Could you check a few things on this model? Use its own coordinates, in mm. A direction names the side the tool comes from. Give positions to 0.01 mm unless a question says otherwise; leave off trailing zeros. Order: outer loops, then holes, each group sorted by start corner. A loop starts at its lowest first (then second) coordinate and runs counter-clockwise, first axis right, second up.
(1) Imagine slicing it at B-B, the plane y = 9.5. Write out the boundary of the cut face in (x, z), then the cut area to 3 significant figures.
(2) If we mould it in two halves opening along Y, with no side actions, what happens to faces 4 (the flat face through (22, -0.8, -3)), 5 (the flat face through (22, 0, -3)), 6 (the flat face through (22, 25, 0.8)), 7 (the flat face through (22, 50, -3))? For each: released by +Y, released by -Y, zero draft, split by the parting line, or undercut.
(3) If I drill on probe 1 along X at (y, z) = (32.5, -3.05); probe 2 along X at (y, z) = (17, -0.4); probe 3 along Y at (x, z) = (36, -1.8), over which ranges is the centre line in solid material (lowest first)?
(4) Will this pin go through, and if not, where does the flat tip stop? pin 1 (1 mm diameter, centred on x = 27, y = 7.5, fed in from -Z).
(5) Imagine slicing it at A-A, the plane z = -2.5. Write out the boundary of the cut face in (x, y).
(6) On a 3-axis mill with a long thin cutter (end or side, diameter ignored), from which of +Z, -Z, +X, -X, +Y, -Y can I reach the whole of each face in a straight line? I mean faces 1 (the flat face through (45.8, 25, -3)), 2 (the cylindrical face through (33.5, 50.4, -3.1)), 3 (the flat face through (45, 25, -3)). Say none if no direction works.
(7) Imagine slicing it at C-C, the plane x = 33.5. Write out the boundary of the cut face in (y, z), then the cut area to 3 significant figures.
from build123d import *

# Parameters (mm, degrees)
F0_W     = 46.6
F0_H     = 51.6
F0_W_2   = 45
F0_H_2   = 50
F1_DEPTH = 0.8
F2_DEPTH = 5
F4_DEPTH = 0.8
F5_R     = 1


with BuildPart() as f1:
    # F0 (on Top) → F1 (new body)
    with BuildSketch(Plane.XY):
        with Locations((22.5, 25)):
            Rectangle(F0_W, F0_H)
        with Locations((22.5, 25)):
            Rectangle(F0_W_2, F0_H_2, mode=Mode.SUBTRACT)
        with Locations((22.5, 25)):
            Rectangle(F0_W_2, F0_H_2)
    extrude(amount=F1_DEPTH)

    # F0 (on Top) → F2 (join)
    with BuildSketch(Plane.XY):
        with Locations((22.5, 25)):
            Rectangle(F0_W, F0_H)
        with Locations((22.5, 25)):
            Rectangle(F0_W_2, F0_H_2, mode=Mode.SUBTRACT)
    extrude(amount=-F2_DEPTH)

    # F3 (on face) → F4 (cut, through all)
    with BuildSketch(Plane(origin=(0, 50.8, 0), x_dir=(-1, 0, 0), z_dir=(0, 1, 0))):
        with BuildLine():
            Line((-35.47274, -5), (-31.67274, -5))
            ThreePointArc((-31.67274, -5), (-33.57274, -3.1), (-35.47274, -5))
        make_face()
        with BuildLine():
            ThreePointArc((-35.47274, -5), (-33.57274, -6.9), (-31.67274, -5))
            Line((-31.67274, -5), (-35.47274, -5))
        make_face()
    extrude(amount=-F4_DEPTH, mode=Mode.SUBTRACT)

    # F5
    f5_edges = [f1.edges().sort_by_distance(p)[0] for p in [
        (-0.8, 25, 0.8),
        (22.5, -0.8, 0.8),
        (45.8, 25, 0.8),
        (22.5, 50.8, 0.8),
        (-0.8, 50.8, -2.1),
        (45.8, 50.8, -2.1),
        (-0.8, -0.8, -2.1),
        (45.8, -0.8, -2.1),
        (22.5, 0, 0),
        (0, 25, 0),
        (22.5, 50, 0),
        (45, 25, 0),
    ]]
    fillet(f5_edges, radius=F5_R)


solid = f1.part
Answer block:
1. outline: (-0.8, -5) - (0, -5) - (0, -1) arc R1 cw to (1, 0) - (44, 0) arc R1 cw to (45, -1) - (45, -5) - (45.8, -5) - (45.8, -0.2) arc R1 ccw to (44.8, 0.8) - (0.2, 0.8) arc R1 ccw to (-0.8, -0.2) - close
1. area: 45.3 mm2
2. face 4: released by -Y
2. face 5: undercut
2. face 6: zero draft
2. face 7: undercut
3. probe 1: x = -0.8 to 0, 45 to 45.8
3. probe 2: x = -0.8 to 0.2, 44.8 to 45.8
3. probe 3: y = -0.8 to 0, 50 to 50.8
4. pin 1: stops at z = 0
5. outline: (-0.8, 0.2) arc R1 ccw to (0.2, -0.8) - (44.8, -0.8) arc R1 ccw to (45.8, 0.2) - (45.8, 49.8) arc R1 ccw to (44.8, 50.8) - (0.2, 50.8) arc R1 ccw to (-0.8, 49.8) - close; hole (0, 0) - (45, 0) - (45, 50) - (0, 50) - close
6. face 1: +Z, -Z, +X, +Y, -Y
6. face 2: -Z, +Y
6. face 3: -Z
7. outline: (-0.8, -5) - (0, -5) - (0, -1) arc R1 cw to (1, 0) - (49, 0) arc R1 cw to (50, -1) - (50, -3.1) - (50.8, -3.1) - (50.8, -0.2) arc R1 ccw to (49.8, 0.8) - (0.2, 0.8) arc R1 ccw to (-0.8, -0.2) - close
7. area: 47.8 mm2
